Answer from the drawing. Dimensions are ordinates in mm from the lowest x, y and z of the part. A direction names the side the tool comes from. Give positions to 0.01 mm unless a question says otherwise; leave off trailing zeros. Write each loop counter-clockwise with the first axis right and the second up, starting at its lowest first coordinate (ties: lowest second). Pieces come first, ordered by that corner, then holes.
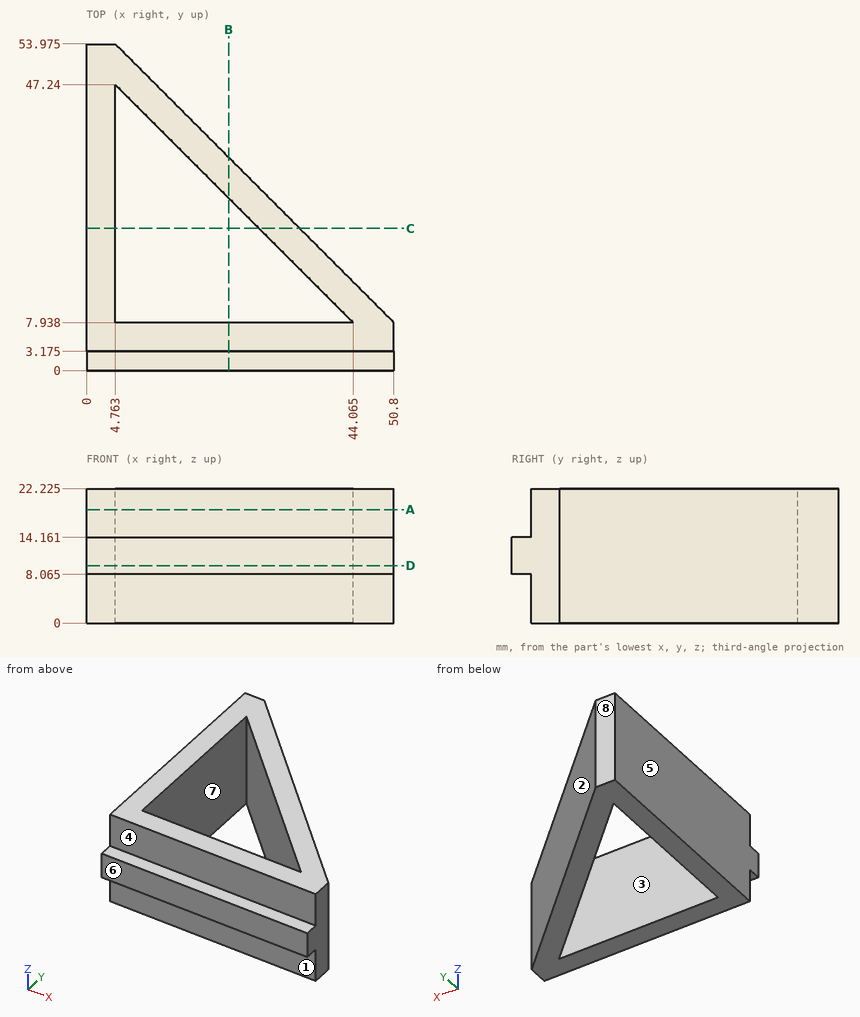
Item 1: Each of these flat-tipped pins is pushed along its axis until it touches: pin 1 Ø6.5 at (x, z) = (14.5, 4.5) entering from -Y (1 decimal); pin 2 Ø1.5 at (x, z) = (23.5, 8.5) entering from +Y; pin 3 Ø8 at (y, z) = (26, 19.5) entering from +X. Where does it stop, or does it pass through?
Result set:
pin 1: stops at y = 3.2
pin 2: stops at y = 35.99
pin 3: stops at x = 36.74
Item 2: Find the intervals of material crossed by line 1 along Y through (x, z) = (29.5, 12.5) (1 decimal); line 2 along Y through (x, z) = (15, 17.5) (1 decimal); line 3 along Y through (x, z) = (2, 15.5) (1 decimal), in increasing order.
Result set:
line 1: y = 0 to 7.9, 22.5 to 29.2
line 2: y = 3.2 to 7.9, 37 to 43.7
line 3: y = 3.2 to 54
Item 3: Section A-A (z = 18.75) is taken. Write down the section's boundary in (x, y) (1 decimal).
Result set:
outline: (0, 3.2) - (50.8, 3.2) - (50.8, 7.9) - (4.8, 54) - (0, 54) - close; hole (4.8, 7.9) - (44.1, 7.9) - (4.8, 47.2) - close
Item 4: Section B-B (x = 23.5) is taken. Write down the section's boundary in (y, z) (1 decimal).
Result set:
outline: (0, 8.1) - (3.2, 8.1) - (3.2, 0) - (7.9, 0) - (7.9, 22.2) - (3.2, 22.2) - (3.2, 14.2) - (0, 14.2) - close; (28.5, 0) - (35.2, 0) - (35.2, 22.2) - (28.5, 22.2) - close
Item 5: Determine the mould class of the marked faces 5, 6, 7 and 8 for opening direction Y: pulls with the +Y half, pulls with the -Y half, needs draft (parallel to the pull), parting line crosses it, or undercut.
Result set:
face 5: needs draft
face 6: pulls with the -Y half
face 7: undercut
face 8: pulls with the +Y half
Item 6: Which of the six approach directions +Z, -Z, +X, -X, +Y, -Y give full straight-line access (tool end or side, diameter ignored) to the marked faces 1, 2, 3 and 4?
Result set:
face 1: -Z, +X, -X, -Y
face 2: +Z, -Z, +X, +Y
face 3: +Z, -Z
face 4: +Z, +X, -X, -Y
Item 7: Section C-C (y = 23.5) is taken. Write down the section's boundary in (x, z) (1 decimal).
Result set:
outline: (0, 0) - (4.8, 0) - (4.8, 22.2) - (0, 22.2) - close; (28.5, 0) - (35.2, 0) - (35.2, 22.2) - (28.5, 22.2) - close
Item 8: Section D-D (z = 9.5) is taken. Write down the section's boundary in (x, y) (1 decimal), and give its area (3 significant figures).
Result set:
outline: (0, 0) - (50.8, 0) - (50.8, 7.9) - (4.8, 54) - (0, 54) - close; hole (4.8, 7.9) - (44.1, 7.9) - (4.8, 47.2) - close
area: 910 mm2
